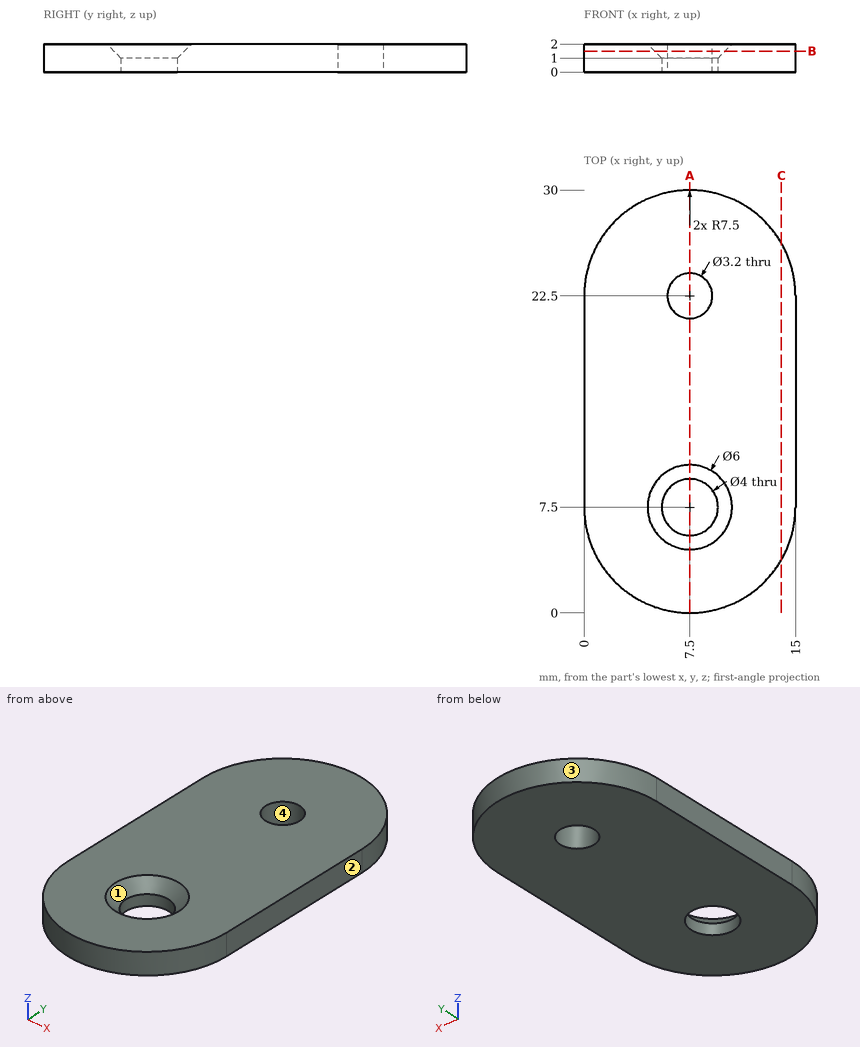
The figure shows three views and two pictorial views of one solid part (mm, origin at its lowest corner). Answer the questions. Coordinates: 2 decimals unless noted, no trailing zeros. Loops run counter-clockwise (first coordinate to the right, second up) from the corner with the lowest first, then second, coordinate; pieces in that order, holes last. Notation, with made-up numbers: (79.5, 57) - (116.5, 57) arc R8 cw to (116.5, 61) - close; hole circle Ø10 at (69.25, 69.5). An arc over 180 degrees is marked (long way). Use a Markdown table: item, result. Add a question column.
1) The part is cut by section C-C, the plane x = 14. Give the vertices of the cut face in (y, z), and give its area (3 significant figures).
2) The part is cut by section A-A, the plane x = 7.5. Give the vertices of the cut face in (y, z).
3) Given pin 1 (3 mm diameter, centred on x = 7.5, y = 22.5, fed in from -Z), flat-ended and moving along its own axis, determine where the tip first touches the part or whether it passes through.
4) The mould has two halves that part along Y. Classify the marked faces 1, 2, 3 and 4: released by +Y, released by -Y, zero draft, split by the parting line, or undercut.
5) The part is cut by section B-B, the plane z = 1.5. Give the vertices of the cut face in (x, y), and give its area (3 significant figures).
6) Find the intervals of material crossed by line 1 (Y direction, x = 7.5, z = 0.5); line 2 (Y direction, x = 7.5, z = 1.55); line 3 (X direction, y = 21.75, z = 1.1), in increasing order.
Here are the results:
| question | item | result |
|---|---|---|
| 1 | outline | (3.76, 0) - (26.24, 0) - (26.24, 2) - (3.76, 2) - close |
| 1 | area | 45.0 mm^2 |
| 2 | outline | (0, 0) - (5.5, 0) - (5.5, 1) - (4.5, 2) - (0, 2) - close; (9.5, 0) - (20.9, 0) - (20.9, 2) - (10.5, 2) - (9.5, 1) - close; (24.1, 0) - (30, 0) - (30, 2) - (24.1, 2) - close |
| 3 | pin 1 | passes through |
| 4 | face 1 | undercut |
| 4 | face 2 | zero draft |
| 4 | face 3 | released by +Y |
| 4 | face 4 | undercut |
| 5 | outline | (0, 7.5) arc R7.5 ccw to (15, 7.5) - (15, 22.5) arc R7.5 ccw to (0, 22.5) - close; hole circle Ø5 at (7.5, 7.5); hole circle Ø3.2 at (7.5, 22.5) |
| 5 | area | 374 mm^2 |
| 6 | line 1 | y = 0 to 5.5, 9.5 to 20.9, 24.1 to 30 |
| 6 | line 2 | y = 0 to 4.95, 10.05 to 20.9, 24.1 to 30 |
| 6 | line 3 | x = 0 to 6.09, 8.91 to 15 |
